Answer from the drawing. Dimensions are ordinates in mm from the lowest x, y and z of the part. A direction names the side the tool comes from. Coordinates: 2 decimals unless noted, no trailing zeros. Write each loop counter-clockwise with the first axis right and the second up, starting at its lowest first coordinate (ties: lowest second). Pieces come first, ordered by that corner, then holes. Notation, with made-up numbers: (-32, 50) -> (15, 50) arc R17 ccw to (15, 68) -> close; hole circle Ø1 at (41, 56). An arc over 180 degrees is marked (long way). One line per item, written item: value. Start each with the question number.
1. Find section D-D, the plane y = 0.9. Write down the section's boundary in (x, z).
2. Given P1, Ø0.8, axis at x = 1.5, z = 7, coming from the -Y side; P2, Ø0.5, axis at x = 3, y = 1, coming from the +Z side, each flat-ended and moving along its own axis, determine where each tip first touches the part or whether it passes through.
3. Find section C-C, the plane x = 1.3. Write down the section's boundary in (y, z).
4. Find section A-A, the plane x = 3.6. Write down the section's boundary in (y, z), and give its area (3 significant figures).
5. Find section B-B, the plane z = 4. Write down the section's boundary in (x, y).
6. For the marked faces 1 and 2, determine the directions among +Z, -Z, +X, -X, +Y, -Y from which every point of the face is accessible in a straight line to the end or side of a thin tool.
7. Consider line 1 along Y through (x, z) = (2.1, 7); line 2 along Z through (x, y) = (2.5, 1.3); line 3 along Y through (x, z) = (0.4, 4.25). Determine where each line is inside the solid, lowest interval first.
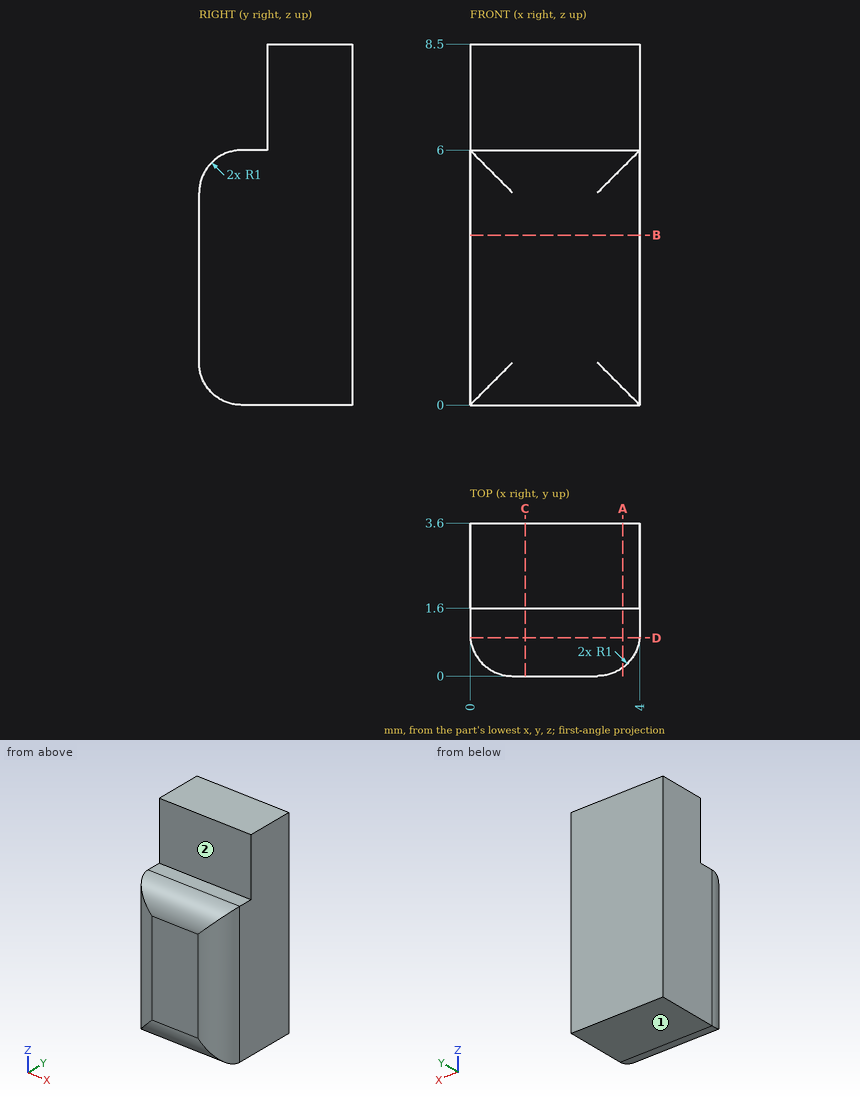
Answer block:
1. outline: (0.01, 0.01) -> (3.99, 0.01) -> (3.99, 5.99) -> (0.01, 5.99) -> close
2. P1: stops at y = 1.6
2. P2: stops at z = 6
3. outline: (0, 1) arc R1 ccw to (1, 0) -> (3.6, 0) -> (3.6, 8.5) -> (1.6, 8.5) -> (1.6, 6) -> (1, 6) arc R1 ccw to (0, 5) -> close
4. outline: (0.2, 0.4) arc R1 ccw to (1, 0) -> (3.6, 0) -> (3.6, 8.5) -> (1.6, 8.5) -> (1.6, 6) -> (1, 6) arc R1 ccw to (0.2, 5.6) -> close
4. area: 25.2 mm2
5. outline: (0, 1) arc R1 ccw to (1, 0) -> (3, 0) arc R1 ccw to (4, 1) -> (4, 3.6) -> (0, 3.6) -> close
6. face 1: -Z, +X, -X, +Y, -Y
6. face 2: +Z, +X, -X, -Y
7. line 1: y = 1.6 to 3.6
7. line 2: z = 0 to 6
7. line 3: y = 0.2 to 3.6
